Could you check a few things on this model? Use its own coordinates, in mm. A direction names the side the tool comes from. Round coordinates to 2 decimals unless told otherwise and drop trailing zeros. Order: outer loops, then holes, each group sorted by start corner. A loop starts at its lowest first (then second) coordinate and runs counter-clockwise, first axis right, second up. Notation, with made-up numbers: (89, -27) -> (132, -27) arc R16 ccw to (132, -15) -> close; hole circle Ø7 at (51, 45). An arc over 180 degrees is marked (long way). One line per question, with ' | ' between items.
```python
from build123d import *

# Parameters (mm, degrees)
SKETCH1_W                                           = 30
SKETCH1_H                                           = 30
BOSS_EXTRUDE1_DEPTH                                 = 7.62
BOSS_EXTRUDE2_DEPTH                                 = 16.75
CUT_EXTRUDE2_DEPTH                                  = 35.39570322
SKETCH3_W                                           = 30
SKETCH3_H                                           = 3.81
BOSS_EXTRUDE3_DEPTH                                 = 10
CSK_FOR_M3_COUNTERSUNK_FLAT_HEAD_SCREW1_D           = 3.4
CSK_FOR_M3_COUNTERSUNK_FLAT_HEAD_SCREW1_CSINK_D     = 6.3
CSK_FOR_M3_COUNTERSUNK_FLAT_HEAD_SCREW1_CSINK_ANGLE = 90
CUT_EXTRUDE3_START                                  = -10
CUT_EXTRUDE3_DEPTH                                  = 52.123313339
SKETCH6_W                                           = 30
SKETCH6_H                                           = 5
CUT_EXTRUDE5_DEPTH                                  = 3.81
FILLET1_R                                           = 1


with BuildPart() as part:
    # Sketch1 → Boss-Extrude1 (new body)
    with BuildSketch(Plane(origin=(0, 0, 0), x_dir=(1, 0, 0), z_dir=(0, 1, 0))):
        Rectangle(SKETCH1_W, SKETCH1_H)
    extrude(amount=BOSS_EXTRUDE1_DEPTH)

    # Sketch2 → Boss-Extrude2 (add)
    with BuildSketch(Plane(origin=(15, 0, 0), x_dir=(0, 0, -1), z_dir=(1, 0, 0))):
        with BuildLine():
            Line((-7.62, 7.62), (-5.08, 7.62))
            ThreePointArc((-5.08, 7.62), (0, 2.54), (5.08, 7.62))
            Line((5.08, 7.62), (7.62, 7.62))
            ThreePointArc((7.62, 7.62), (0, 0), (-7.62, 7.62))
        make_face()
    boss_extrude2 = extrude(amount=BOSS_EXTRUDE2_DEPTH)

    # Sketch2<4> → Cut-Extrude2 (cut, through all)
    with BuildSketch(Plane(origin=(15, 0, 0), x_dir=(0, 0, -1), z_dir=(1, 0, 0))):
        with BuildLine():
            Line((5.08, 7.62), (-5.08, 7.62))
            ThreePointArc((-5.08, 7.62), (0, 2.54), (5.08, 7.62))
        make_face()
    extrude(amount=-CUT_EXTRUDE2_DEPTH, mode=Mode.SUBTRACT)

    # Mirror1: Boss-Extrude2 across plane
    add(boss_extrude2.mirror(Plane(origin=(0, 0, 0), x_dir=(0, 0, 1), z_dir=(1, 0, 0))))

    # Sketch3 → Boss-Extrude3 (add)
    with BuildSketch(Plane.XY.offset(15)):
        with Locations((0, 5.715)):
            Rectangle(SKETCH3_W, SKETCH3_H)
    boss_extrude3 = extrude(amount=BOSS_EXTRUDE3_DEPTH)

    # CSK for M3 Countersunk Flat Head Screw1 (through all)
    with Locations(Plane(origin=(0, 3.81, 19.31), x_dir=(0, 0, -1), z_dir=(0, -1, 0))):
        with Locations((0, 0)):
            csk_for_m3_countersunk_flat_head_screw1 = CounterSinkHole(CSK_FOR_M3_COUNTERSUNK_FLAT_HEAD_SCREW1_D / 2, CSK_FOR_M3_COUNTERSUNK_FLAT_HEAD_SCREW1_CSINK_D / 2, counter_sink_angle=CSK_FOR_M3_COUNTERSUNK_FLAT_HEAD_SCREW1_CSINK_ANGLE)

    # Sketch4 → Cut-Extrude3 (cut)
    with BuildSketch(Plane(origin=(0, 7.62, 0), x_dir=(1, 0, 0), z_dir=(0, 1, 0)).offset(CUT_EXTRUDE3_START)):
        with BuildLine():
            Line((-15, -25), (-1.2e-08, -25))
            ThreePointArc((-1.2e-08, -25), (-10.606601722, -20.606601713), (-15, -10))
            Line((-15, -10), (-15, -25))
        make_face()
        with BuildLine():
            Line((15, -25), (15, -10))
            ThreePointArc((15, -10), (10.606601713, -20.606601722), (-1.2e-08, -25))
            Line((-1.2e-08, -25), (15, -25))
        make_face()
    cut_extrude3 = extrude(amount=CUT_EXTRUDE3_DEPTH, mode=Mode.SUBTRACT)

    # Mirror2: Boss-Extrude3, CSK for M3 Countersunk Flat Head Screw1, Cut-Extrude3 across plane
    add(boss_extrude3.mirror(Plane.XY))
    add(csk_for_m3_countersunk_flat_head_screw1.mirror(Plane.XY), mode=Mode.SUBTRACT)
    add(cut_extrude3.mirror(Plane.XY), mode=Mode.SUBTRACT)

    # Sketch6 → Cut-Extrude5 (cut)
    with BuildSketch(Plane.XZ):
        with Locations((0, 12.5)):
            Rectangle(SKETCH6_W, SKETCH6_H)
        with Locations((0, -12.5)):
            Rectangle(SKETCH6_W, SKETCH6_H)
    extrude(amount=-CUT_EXTRUDE5_DEPTH, mode=Mode.SUBTRACT)

    # Fillet1
    # the kernel refuses this fillet: 1 mm, written as the material it adds along each edge
    with BuildSketch(Plane(origin=(-17.5, 3.81, 10), x_dir=(0, 0, 1), z_dir=(1, 0, 0))) as fillet1_piece_1_section:
        with BuildLine():
            CenterArc((FILLET1_R, FILLET1_R), FILLET1_R, 180, 90)
            Line((0, FILLET1_R), (0, 0))
            Line((0, 0), (FILLET1_R, 0))
        make_face()
    fillet1_piece_1 = extrude(amount=35, mode=Mode.PRIVATE)
    fillet1_piece_1 = fillet1_piece_1 & Plane(origin=(0, 3.58660625, 10), x_dir=(-8.322182034394214e-10, 0, 1.0), z_dir=(0, -1, 0)) * Cylinder(15, 74, mode=Mode.PRIVATE)
    add(fillet1_piece_1)
    with BuildSketch(Plane(origin=(-17.5, 3.81, -10), x_dir=(0, 0, -1), z_dir=(1, 0, 0))) as fillet1_piece_2_section:
        with BuildLine():
            CenterArc((FILLET1_R, -FILLET1_R), FILLET1_R, 90, 90)
            Line((0, -FILLET1_R), (0, 0))
            Line((0, 0), (FILLET1_R, 0))
        make_face()
    fillet1_piece_2 = extrude(amount=35, mode=Mode.PRIVATE)
    fillet1_piece_2 = fillet1_piece_2 & Plane(origin=(0, 3.586606238, -10), x_dir=(1, 0, 0), z_dir=(0, -1, 0)) * Cylinder(15, 74, mode=Mode.PRIVATE)
    add(fillet1_piece_2)
    # the kernel refuses this fillet: 1 mm, written as the material it takes off along each edge
    with BuildSketch(Plane(origin=(-17.5, 0, 10), x_dir=(0, 1, 0), z_dir=(1, 0, 0)), Plane(origin=(-17.5, 0, -10), x_dir=(0, 0, 1), z_dir=(1, 0, 0))) as fillet1_2_piece_1:
        with BuildLine():
            CenterArc((FILLET1_R, -FILLET1_R), FILLET1_R, 90, 90)
            Line((0, -FILLET1_R), (0, 0))
            Line((0, 0), (FILLET1_R, 0))
        make_face()
    extrude(amount=35, mode=Mode.SUBTRACT)


solid = part.part
```
1. On a 3-axis mill with a long thin cutter (end or side, diameter ignored), from which of +Z, -Z, +X, -X, +Y, -Y can I reach the whole of each face in a straight line? I mean faces 4 (the face through (15, 3, -7)), 5 (the face through (0, 2, -10)), 6 (the face through (23, 0, 0)). Say none if no direction works.
From the geometry:
face 4: -Z, +X, -Y | face 5: -Z, +X, -X, -Y | face 6: +X, -Y
2. I want a section at D-D on x = -7. List the corners of the cut face in (y, z) for me.
From the geometry:
outline: (0, -9) arc R1 ccw to (1, -10) -> (2.81, -10) arc R1 cw to (3.81, -11) -> (3.81, -23.27) -> (7.62, -23.27) -> (7.62, -5.08) arc R5.08 cw to (7.62, 5.08) -> (7.62, 23.27) -> (3.81, 23.27) -> (3.81, 11) arc R1 cw to (2.81, 10) -> (1, 10) arc R1 ccw to (0, 9) -> close
3. I need wall thicknesses on probe 1 along Z at (x, y) = (0, 6.4); probe 2 along Z at (x, y) = (0, 6.9); probe 3 along X at (y, z) = (3, -8.5). Which ranges of each line are inside material? Lowest first, please.
From the geometry:
probe 1: z = -25 to -21.01, -17.61 to -4.93, 4.93 to 17.61, 21.01 to 25 | probe 2: z = -25 to -21.01, -17.61 to -5.03, 5.03 to 17.61, 21.01 to 25 | probe 3: x = -15 to 15
4. I want a section at B-B on x = 5.5. List the corners of the cut face in (y, z) for me.
From the geometry:
outline: (0, -9) arc R1 ccw to (1, -10) -> (2.81, -10) arc R1 cw to (3.81, -11) -> (3.81, -23.96) -> (7.62, -23.96) -> (7.62, -5.08) arc R5.08 cw to (7.62, 5.08) -> (7.62, 23.96) -> (3.81, 23.96) -> (3.81, 11) arc R1 cw to (2.81, 10) -> (1, 10) arc R1 ccw to (0, 9) -> close
5. I want a section at C-C on z = -6. List the corners of the cut face in (x, y) for me, and give its area (3 significant figures).
From the geometry:
outline: (-31.75, 2.92) -> (-15, 2.92) -> (-15, 0) -> (15, 0) -> (15, 2.92) -> (31.75, 2.92) -> (31.75, 7.62) -> (-31.75, 7.62) -> close | area: 386 mm²
6. I want a section at A-A on z = 19.31. List the corners of the cut face in (x, y) for me.
From the geometry:
outline: (-11.76, 3.81) -> (-3.15, 3.81) -> (-1.7, 5.26) -> (-1.7, 7.62) -> (-11.76, 7.62) -> close; (1.7, 5.26) -> (3.15, 3.81) -> (11.76, 3.81) -> (11.76, 7.62) -> (1.7, 7.62) -> close
7. I'm going to push flat-ended pins straight in: pin 1 (12 mm diameter, centred on x = 17, z = 10.5, fed in from -Y); pin 2 (0.5 mm diameter, centred on x = -6.5, y = 1.5, fed in from +Z); pin 3 (2 mm diameter, centred on y = 1, z = -10, fed in from -X); pin 4 (1.5 mm diameter, centred on y = 1, z = 11, fed in from -X). Where does each tip first touch, or does it pass through?
From the geometry:
pin 1: stops at y = 0 | pin 2: stops at z = 10 | pin 3: stops at x = -15 | pin 4: passes through
8. If we mould it in two halves opening along X, with no side actions, what happens to faces 1 (the face through (-15, 3, 7)), 2 (the face through (0, 2, 10)), 3 (the face through (0.07, 6.46, -17.61))? For each: pulls with the +X half, pulls with the -X half, needs draft (parallel to the pull), parting line crosses it, or undercut.
From the geometry:
face 1: pulls with the -X half | face 2: needs draft | face 3: undercut
